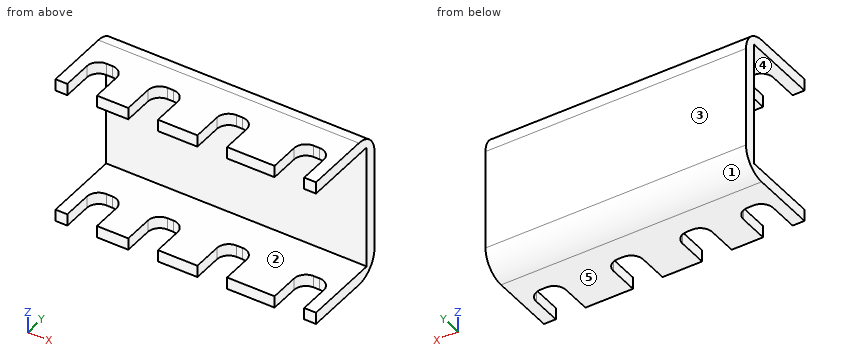
```python
from build123d import *

# Parameters (mm, degrees)
ESBO_O1_W                = 44
ESBO_O1_H                = 25
RESSALTO_EXTRUS_O1_DEPTH = 7.5
CASCA1_T                 = -2
ESBO_O2_W                = 5
ESBO_O2_H                = 14
CORTE_EXTRUS_O1_DEPTH    = 35.135758377
FILETE1_R                = 2
FILETE2_R                = 4


with BuildPart() as part:
    # Esboço1 → Ressalto-extrusão1 (new, symmetric)
    with BuildSketch(Plane(origin=(0, 0, 0), x_dir=(1, 0, 0), z_dir=(0, 1, 0))):
        Rectangle(ESBO_O1_W, ESBO_O1_H)
    extrude(amount=RESSALTO_EXTRUS_O1_DEPTH, both=True)

    # Casca1
    casca1_openings = [part.faces().sort_by_distance(p)[0] for p in [
        (0, -7.5, 0),
        (-22, 0, 0),
        (22, 0, 0),
    ]]
    offset(amount=CASCA1_T, openings=casca1_openings, kind=Kind.INTERSECTION)

    # Esboço2 → Corte-extrusão1 (cut, through all)
    with BuildSketch(Plane.XY.offset(12.5)):
        with Locations((-7.203332481, -7.5)):
            Rectangle(ESBO_O2_W, ESBO_O2_H)
        with Locations((-17.5, -7.5)):
            Rectangle(ESBO_O2_W, ESBO_O2_H)
        with Locations((4.47023527, -7.5)):
            Rectangle(ESBO_O2_W, ESBO_O2_H)
        with Locations((17.5, -7.5)):
            Rectangle(ESBO_O2_W, ESBO_O2_H)
    extrude(amount=-CORTE_EXTRUS_O1_DEPTH, mode=Mode.SUBTRACT)

    # Filete1
    filete1_edges = [part.edges().sort_by_distance(p)[0] for p in [
        (20, -0.5, -11.5),
        (15, -0.5, -11.5),
        (20, -0.5, 11.5),
        (15, -0.5, 11.5),
        (-15, -0.5, -11.5),
        (-20, -0.5, -11.5),
        (-15, -0.5, 11.5),
        (-20, -0.5, 11.5),
        (-4.703332481, -0.5, -11.5),
        (-9.703332481, -0.5, -11.5),
        (-4.703332481, -0.5, 11.5),
        (-9.703332481, -0.5, 11.5),
        (6.97023527, -0.5, -11.5),
        (1.97023527, -0.5, -11.5),
        (6.97023527, -0.5, 11.5),
        (1.97023527, -0.5, 11.5),
    ]]
    fillet(filete1_edges, radius=FILETE1_R)

    # Filete2
    filete2_edges = [part.edges().sort_by_distance(p)[0] for p in [
        (0, 7.5, 12.5),
        (0, 7.5, -12.5),
    ]]
    fillet(filete2_edges, radius=FILETE2_R)


solid = part.part
```
Input: part model. Units: mm. Frame: model coordinates. Face numbers are marked on the shaded views. A direction names the side the tool comes from. Coordinates: 2 decimals unless noted, no trailing zeros. Loops run counter-clockwise (first coordinate to the right, second up) from the corner with the lowest first, then second, coordinate; pieces in that order, holes last. Notation, with made-up numbers: M -2.75,18.25 L 31.25,18.25 A11 ccw 31.25,25.25 Z; hole C 41,-31 d2. An arc over 180 degrees is marked long. Use a Markdown table: item, result. Add a question column.
1) Line query: L1, parallel to Z at x = 2.5, y = 3; L2, parallel to X at y = -4.25, z = 10.75; L3, parallel to Y at x = 8, z = -6.5. Output: solid intervals per line, ascending. Write a range as from..to.
2) Section B-B, the plane x = 17.5. Return the cut outline in (y, z), plus the area to 3 significant figures.
3) Section D-D, the plane y = -3. Give the number of separate pieces and of enclosed holes in the cut face, plus the area to 3 significant figures.
4) Set-up query: the marked faces 4 and 5. Return all of +Z, -Z, +X, -X, +Y, -Y with unobstructed straight access to the full face (end or side cutting, diameter ignored); none if empty.
5) Section A-A, the plane y = 0.5. Return the cut outline in (x, z), plus the area to 3 significant figures.
6) Pin query (flat end, axial travel): P1, Ø1.1, axis at x = 17.5, z = 11.5, coming from the -Y side; P2, Ø10, axis at x = -0.5, z = 0.5, coming from the -Y side; P3, Ø1, axis at x = -17.5, y = 6, coming from the -Z side. Return the tip coordinate at first contact, or that it passes through.
7) Section C-C, the plane z = -2. Return the cut outline in (x, y).
8) Draft query along Z for the marked faces 1, 2 and 3. Return one class per face: +Z half, -Z half, draft (parallel to the pull), parting line (faces both ways), or undercut.
Answer below:
| question | item | result |
|---|---|---|
| 1 | L1 | -12.5..-10.5, 10.5..12.5 |
| 1 | L2 | -22..-20, -15..-9.7, -4.7..1.97, 6.97..15, 20..22 |
| 1 | L3 | 5.5..7.5 |
| 2 | outline | M -0.5,-12.5 L 3.5,-12.5 A4 ccw 7.5,-8.5 L 7.5,8.5 A4 ccw 3.5,12.5 L -0.5,12.5 L -0.5,10.5 L 5.5,10.5 L 5.5,-10.5 L -0.5,-10.5 Z |
| 2 | area | 67.1 mm2 |
| 3 | separate pieces | 10 |
| 3 | enclosed holes | 0 |
| 3 | area | 96.0 mm2 |
| 4 | face 4 | +X, -X, -Y |
| 4 | face 5 | -Z, +X, -X, +Y, -Y |
| 5 | outline | M -22,-12.5 L 22,-12.5 L 22,-10.5 L -22,-10.5 Z; M -22,10.5 L 22,10.5 L 22,12.5 L -22,12.5 Z |
| 5 | area | 176 mm2 |
| 6 | P1 | y = -0.5 |
| 6 | P2 | y = 5.5 |
| 6 | P3 | z = -11.96 |
| 7 | outline | M -22,5.5 L 22,5.5 L 22,7.5 L -22,7.5 Z |
| 8 | face 1 | -Z half |
| 8 | face 2 | undercut |
| 8 | face 3 | draft |
